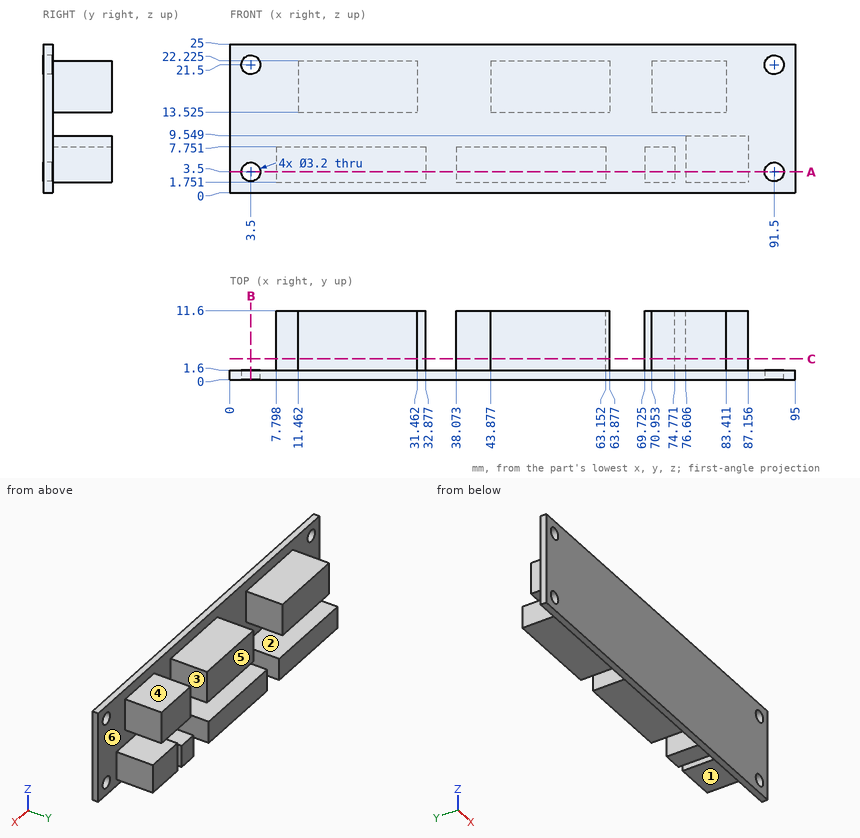
Source: three-view drawing plus pictorial views. Frame: mm from the lowest corner of the part. A direction names the side the tool comes from. Round coordinates to 2 decimals unless told otherwise and drop trailing zeros. Write each loop counter-clockwise with the first axis right and the second up, starting at its lowest first coordinate (ties: lowest second). Pieces come first, ordered by that corner, then holes. Notation, with made-up numbers: M 75.25,-31.75 L 119.25,-31.75 A24 cw 119.25,3.25 Z; hole C -12,41 d10. An arc over 180 degrees is marked long. One line per item, written item: value. Start each with the question number.
Item 1: Mould query, pull axis Z, two halves, no side actions, for the marked faces 4, 5 and 6. Classes: pulls with the +Z half, pulls with the -Z half, needs draft (parallel to the pull), parting line crosses it, or undercut.
Item 2: Set-up query: the marked faces 1, 2 and 3. Return all of +Z, -Z, +X, -X, +Y, -Y with unobstructed straight access to the full face (end or side cutting, diameter ignored); none if empty.
Item 3: Section query A-A (z = 3.5). Return the cut outline in (x, y) (1 decimal).
Item 4: Ray query, L1, parallel to X at y = 7, z = 7.5 (1 decimal); L2, parallel to X at y = 1.2, z = 21.5; L3, parallel to Z at x = 3.5, y = 1.05. Return the intervals inside material, ascending. Write a range as from..to.
Item 5: Section query C-C (y = 3.5). State how many separate pieces and enclosed holes the cut face has, plus the area to 3 significant figures.
Item 6: Pin query (flat end, axial travel): pin 1 (3 mm diameter, centred on y = 9, z = 9.5, fed in from -X) (1 decimal); pin 2 (2.5 mm diameter, centred on y = 5, z = 20, fed in from +X); pin 3 (6.5 mm diameter, centred on y = 6, z = 6, fed in from +X). Return the tip coordinate at first contact, or that it passes through.
Item 7: Section query B-B (x = 3.5). Return the cut outline in (y, z).
Result set:
1. face 4: pulls with the +Z half
1. face 5: needs draft
1. face 6: undercut
2. face 1: -Z, +X, -X, +Y
2. face 2: -X, +Y
2. face 3: +Z, -Z, +Y
3. outline: M 0,0 L 1.9,0 L 1.9,1.6 L 0,1.6 Z; M 5.1,0 L 89.9,0 L 89.9,1.6 L 87.2,1.6 L 87.2,11.6 L 76.6,11.6 L 76.6,1.6 L 74.8,1.6 L 74.8,11.6 L 69.7,11.6 L 69.7,1.6 L 63.2,1.6 L 63.2,11.6 L 38.1,11.6 L 38.1,1.6 L 32.9,1.6 L 32.9,11.6 L 7.8,11.6 L 7.8,1.6 L 5.1,1.6 Z; M 93.1,0 L 95,0 L 95,1.6 L 93.1,1.6 Z
4. L1: x = 7.8..32.9, 38.1..63.2, 69.7..74.8, 76.6..87.2
4. L2: x = 0..1.9, 5.1..89.9, 93.1..95
4. L3: z = 0..1.9, 5.1..19.9, 23.1..25
5. separate pieces: 7
5. enclosed holes: 0
5. area: 870 mm²
6. pin 1: stops at x = 76.6
6. pin 2: stops at x = 83.41
6. pin 3: stops at x = 87.16
7. outline: M 0,0 L 1.6,0 L 1.6,1.9 L 0,1.9 Z; M 0,5.1 L 1.6,5.1 L 1.6,19.9 L 0,19.9 Z; M 0,23.1 L 1.6,23.1 L 1.6,25 L 0,25 Z
